Check sheet for the modelled part. Datum: model origin and axes. Units: mm. Round coordinates to 2 decimals unless told otherwise and drop trailing zeros. Loops run counter-clockwise (first coordinate to the right, second up) from the corner with the lowest first, then second, coordinate; pieces in that order, holes last. Notation, with made-up numbers: (13, 28) -> (28, 28) arc R17 cw to (28, 42) -> close; hole circle Ø5 at (32.25, -39.75). An arc over 180 degrees is marked (long way). Return JSON: item names as keys, results as strings.
Autodesk Inventor part; units mm, degrees
ref_plane "YZ Plane" through (0, 0, 0) normal (1, 0, 0) x (0, 1, 0)
ref_plane "XY Plane" through (0, 0, 0) normal (0, 0, 1) x (1, 0, 0)
sketch "Esquisse1" plane through (0, 0, 0) normal (0, 0, 1) x (1, 0, 0)
  circle A0 centre (0, 0) radius 77.5
  circle A1 centre (0, 0) radius 20
  dimension "d0" = 155
  dimension "d1" = 40
extrude "Extrusion1" add sketch "Esquisse1" against normal blind 5
sketch "Esquisse2" plane through (0, 0, 0) normal (0, 0, 1) x (1, 0, 0)
  circle A0 centre (0, 0) radius 27.5
  line L0 (0, 0) -> (35.9549, 35.9549)
  line L1 (-108.5, 0) -> (108.5, 0)
  point P0 (19.4454, 19.4454)
  dimension "d11" = 55
  dimension "d15" = 45
hole "Perçage1" at (19.4454, 19.4454, 0) direction (0, 0, -1) diameter 6.6 end through all
pattern_circular "Réseau circulaire1" count 4 over 360 about axis through (0, 0, 0) along (0, 0, -1) of "Perçage1"
properties part number "Flasque"
Q1. Section check B-B (y = 4). Record the boundary of the cut face in (x, z), then the cut area to 3 significant figures.
Results list:
{"outline": "(-77.4, -5) -> (-19.6, -5) -> (-19.6, 0) -> (-77.4, 0) -> close; (19.6, -5) -> (77.4, -5) -> (77.4, 0) -> (19.6, 0) -> close", "area": "578 mm^2"}
Q2. Section check A-A (x = 0). Record the boundary of the cut face in (y, z).
Results list:
{"outline": "(-77.5, -5) -> (-20, -5) -> (-20, 0) -> (-77.5, 0) -> close; (20, -5) -> (77.5, -5) -> (77.5, 0) -> (20, 0) -> close"}
Q3. Section check C-C (z = -2.95). Record the boundary of the cut face in (x, y), then the cut area to 3 significant figures.
Results list:
{"outline": "circle Ø155 at (0, 0); hole circle Ø6.6 at (-19.45, -19.45); hole circle Ø6.6 at (-19.45, 19.45); hole circle Ø40 at (0, 0); hole circle Ø6.6 at (19.45, -19.45); hole circle Ø6.6 at (19.45, 19.45)", "area": "17,500 mm^2"}
Q4. Material ranges on line 1 (Y direction, x = 0, z = -1.2); line 2 (Y direction, x = -16.5, z = -1.65); line 3 (X direction, y = -1, z = -1.3), recorded low to high.
Results list:
{"line 1": "-77.5 to -20, 20 to 77.5", "line 2": "-75.72 to -20.93, -17.96 to -11.3, 11.3 to 17.96, 20.93 to 75.72", "line 3": "-77.49 to -19.97, 19.97 to 77.49"}
Q5. Draft check along Y on faces 1 (the flat face through (16, -16, -5)), 2 (the cylindrical face through (-16.8, -75.657, -2.465)), 3 (the cylindrical face through (-19.3, -22.742, -2.535)). Enter one of: released by +Y, released by -Y, zero draft, split by the parting line, or undercut.
Results list:
{"face 1": "zero draft", "face 2": "split by the parting line", "face 3": "undercut"}
Q6. Section check D-D (x = -51). Record the boundary of the cut face in (y, z), then the cut area to 3 significant figures.
Results list:
{"outline": "(-58.35, -5) -> (58.35, -5) -> (58.35, 0) -> (-58.35, 0) -> close", "area": "584 mm^2"}
Q7. Go/stop test with flat-tipped pins: pin 1 (2 mm diameter, centred on x = -12.5, z = -3.5, fed in from +Y); pin 2 (1 mm diameter, centred on x = 16, z = -1.5, fed in from +Y); pin 3 (1 mm diameter, centred on y = -8, z = -2.5, fed in from -X); pin 4 (5.5 mm diameter, centred on x = 19.45, y = 19.45, fed in from +Z). Record where each tip stops, or that it passes through.
Results list:
{"pin 1": "y = 76.64", "pin 2": "y = 75.93", "pin 3": "x = -77.14", "pin 4": "through"}
